Source: CAD feature listing. Evaluate the final solid. Frame: model axes, mm. A direction names the side the tool comes from. Coordinates: 2 decimals unless noted, no trailing zeros.
Item 1: Line query: probe 1 along Z at (x, y) = (60, 2); probe 2 along Z at (x, y) = (99, 2). Output: solid intervals per line, ascending.
Item 2: Pull-direction query (Z, two-part tool) for faces 3 (the cylindrical face through (78.514, 2.896, -19.391)), 4 (the flat face through (0, 3, -30)), 5 (the flat face through (141.4, 2.6, -21.4)); classes: +Z half, -Z half, draft (parallel to the pull), parting line (faces both ways), or undercut.
Item 3: Pin query (flat end, axial travel): pin 1 Ø1 at (y, z) = (2, -21.5) entering from -X; pin 2 Ø2.5 at (x, z) = (99.99, -20.02) entering from +Y (1 decimal); pin 3 Ø5.5 at (x, z) = (140, -39.99) entering from +Y. Return the tip coordinate at first contact, or that it passes through.
Item 4: Reachability of faces 1 (the cylindrical face through (141.652, 1.318, -20.411)), 2 (the cylindrical face through (122.88, 4.31, -18.5)) from +Z, -Z, +X, -X, +Y, -Y: full face, straight path, thin tool, end or side. Return the list, or none.
Item 5: Section query A-A, the plane y = 4.25. State how many separate pieces and enclosed holes the cut face has, then the cut area to 3 significant figures.
```python
from build123d import *

# Parameters (mm, degrees)
SKETCH1_W                      = 160
SKETCH1_H                      = 60
BOSS_EXTRUDE1_DEPTH            = 6
M3_CLEARANCE_HOLE1_D           = 3.4
M3_CLEARANCE_HOLE1_CSINK_D     = 3.45
M3_CLEARANCE_HOLE1_CSINK_ANGLE = 90
M3_CLEARANCE_HOLE3_D           = 3.4
M3_CLEARANCE_HOLE3_CSINK_D     = 3.45
M3_CLEARANCE_HOLE3_CSINK_ANGLE = 90
M3_CLEARANCE_HOLE4_D           = 3.2
M3_CLEARANCE_HOLE4_CSINK_D     = 3.45
M3_CLEARANCE_HOLE4_CSINK_ANGLE = 90
M3_CLEARANCE_HOLE5_D           = 3.2
M3_CLEARANCE_HOLE5_CSINK_D     = 3.45
M3_CLEARANCE_HOLE5_CSINK_ANGLE = 90
CUT_EXTRUDE3_DEPTH             = 171.985379492
CUT_EXTRUDE4_DEPTH             = 171.985379492
CUT_EXTRUDE5_DEPTH             = 171.985379492
CUT_EXTRUDE6_DEPTH             = 171.985379492
CUT_EXTRUDE7_DEPTH             = 171.985379492
CUT_EXTRUDE8_DEPTH             = 171.985379492


with BuildPart() as part:
    # Sketch1 → Boss-Extrude1 (new body)
    with BuildSketch(Plane(origin=(0, 0, 0), x_dir=(1, 0, 0), z_dir=(0, 1, 0))):
        with Locations((80, 30)):
            Rectangle(SKETCH1_W, SKETCH1_H)
    extrude(amount=BOSS_EXTRUDE1_DEPTH)

    # Sketch4 → CBORE for M3 Hex Socket Head Cap Screw1 (revolve, cut)
    with BuildSketch(Plane(origin=(139.992504276, 6, -20.042969634), x_dir=(0, 0, 1), z_dir=(1, 0, 0))):
        Polygon((0, 0), (0, 6), (1.7, 6), (1.7, 3.4), (3.25, 3.4), (3.25, 0.025), (3.275, 0), align=None)
    revolve(axis=Axis((139.992504276, 12.35, -20.042969634), (0, -1, 0)), mode=Mode.SUBTRACT)

    # Sketch7 → CBORE for M3 Hex Socket Head Cap Screw2 (revolve, cut)
    with BuildSketch(Plane(origin=(140.004074622, 6, -39.992947499), x_dir=(0, 0, 1), z_dir=(1, 0, 0))):
        Polygon((0, 0), (0, 6), (1.7, 6), (1.7, 3.4), (3.25, 3.4), (3.25, 0.025), (3.275, 0), align=None)
    revolve(axis=Axis((140.004074622, 12.35, -39.992947499), (0, -1, 0)), mode=Mode.SUBTRACT)

    # Sketch10 → CBORE for M3 Hex Socket Head Cap Screw3 (revolve, cut)
    with BuildSketch(Plane(origin=(120.000202739, 6, -39.984949452), x_dir=(0, 0, 1), z_dir=(1, 0, 0))):
        Polygon((0, 0), (0, 6), (1.6, 6), (1.6, 3.4), (3.25, 3.4), (3.25, 0.025), (3.275, 0), align=None)
    revolve(axis=Axis((120.000202739, 12.35, -39.984949452), (0, -1, 0)), mode=Mode.SUBTRACT)

    # Sketch13 → CBORE for M3 Hex Socket Head Cap Screw4 (revolve, cut)
    with BuildSketch(Plane(origin=(119.997329442, 6, -19.99932447), x_dir=(0, 0, 1), z_dir=(1, 0, 0))):
        Polygon((0, 0), (0, 6), (1.6, 6), (1.6, 3.4), (3.25, 3.4), (3.25, 0.025), (3.275, 0), align=None)
    revolve(axis=Axis((119.997329442, 12.35, -19.99932447), (0, -1, 0)), mode=Mode.SUBTRACT)

    # M3 Clearance Hole1 (through all)
    with Locations(Plane(origin=(0, 6, 0), x_dir=(1, 0, 0), z_dir=(0, 1, 0))):
        with Locations((100.019720451, 40.002637401)):
            CounterSinkHole(M3_CLEARANCE_HOLE1_D / 2, M3_CLEARANCE_HOLE1_CSINK_D / 2, counter_sink_angle=M3_CLEARANCE_HOLE1_CSINK_ANGLE)

    # M3 Clearance Hole3 (through all)
    with Locations(Plane(origin=(0, 6, 0), x_dir=(1, 0, 0), z_dir=(0, 1, 0))):
        with Locations((99.99392625, 20.015973)):
            CounterSinkHole(M3_CLEARANCE_HOLE3_D / 2, M3_CLEARANCE_HOLE3_CSINK_D / 2, counter_sink_angle=M3_CLEARANCE_HOLE3_CSINK_ANGLE)

    # M3 Clearance Hole4 (through all)
    with Locations(Plane(origin=(0, 6, 0), x_dir=(1, 0, 0), z_dir=(0, 1, 0))):
        with Locations((79.997225907, 40.005191988)):
            CounterSinkHole(M3_CLEARANCE_HOLE4_D / 2, M3_CLEARANCE_HOLE4_CSINK_D / 2, counter_sink_angle=M3_CLEARANCE_HOLE4_CSINK_ANGLE)

    # M3 Clearance Hole5 (through all)
    with Locations(Plane(origin=(0, 6, 0), x_dir=(1, 0, 0), z_dir=(0, 1, 0))):
        with Locations((79.991526723, 20.004071528)):
            CounterSinkHole(M3_CLEARANCE_HOLE5_D / 2, M3_CLEARANCE_HOLE5_CSINK_D / 2, counter_sink_angle=M3_CLEARANCE_HOLE5_CSINK_ANGLE)

    # Sketch2 → Cut-Extrude3 (cut, through all)
    with BuildSketch(Plane(origin=(0, 6, 0), x_dir=(1, 0, 0), z_dir=(0, 1, 0))):
        Polygon((61.499825244, 20.000000122), (61.29888673, 20.749912866), (60.7499125, 21.298887096), (59.999999756, 21.49982561), (59.250087012, 21.298887096), (58.701112782, 20.749912866), (58.500174268, 20.000000122), (58.701112782, 19.250087378), (59.250087012, 18.701113148), (59.999999756, 18.500174634), (60.7499125, 18.701113148), (61.29888673, 19.250087378), align=None)
    extrude(amount=-CUT_EXTRUDE3_DEPTH, mode=Mode.SUBTRACT)

    # Sketch35 → Cut-Extrude4 (cut, through all)
    with BuildSketch(Plane(origin=(0, 6, 0), x_dir=(1, 0, 0), z_dir=(0, 1, 0))):
        Polygon((58.500006975, 40), (58.700967935, 39.250003488), (59.250003488, 38.700967935), (60, 38.500006975), (60.749996512, 38.700967935), (61.299032065, 39.250003488), (61.499993025, 40), (61.299032065, 40.749996512), (60.749996512, 41.299032065), (60, 41.499993025), (59.250003488, 41.299032065), (58.700967935, 40.749996512), align=None)
    extrude(amount=-CUT_EXTRUDE4_DEPTH, mode=Mode.SUBTRACT)

    # Sketch36 → Cut-Extrude5 (cut, through all)
    with BuildSketch(Plane(origin=(0, 6, 0), x_dir=(1, 0, 0), z_dir=(0, 1, 0))):
        Polygon((41.5, 20), (41.149066665, 20.964181415), (40.260472267, 21.47721163), (39.25, 21.299038106), (38.590461069, 20.513030215), (38.590461069, 19.486969785), (39.25, 18.700961894), (40.260472267, 18.52278837), (41.149066665, 19.035818585), align=None)
    extrude(amount=-CUT_EXTRUDE5_DEPTH, mode=Mode.SUBTRACT)

    # Sketch37 → Cut-Extrude6 (cut, through all)
    with BuildSketch(Plane(origin=(0, 6, 0), x_dir=(1, 0, 0), z_dir=(0, 1, 0))):
        Polygon((41.5, 40), (41.149066665, 40.964181415), (40.260472267, 41.47721163), (39.25, 41.299038106), (38.590461069, 40.513030215), (38.590461069, 39.486969785), (39.25, 38.700961894), (40.260472267, 38.52278837), (41.149066665, 39.035818585), align=None)
    extrude(amount=-CUT_EXTRUDE6_DEPTH, mode=Mode.SUBTRACT)

    # Sketch38 → Cut-Extrude7 (cut, through all)
    with BuildSketch(Plane(origin=(0, 6, 0), x_dir=(1, 0, 0), z_dir=(0, 1, 0))):
        Polygon((21.5, 20), (20.75, 21.299038106), (19.25, 21.299038106), (18.5, 20), (19.25, 18.700961894), (20.75, 18.700961894), align=None)
    extrude(amount=-CUT_EXTRUDE7_DEPTH, mode=Mode.SUBTRACT)

    # Sketch39 → Cut-Extrude8 (cut, through all)
    with BuildSketch(Plane(origin=(0, 6, 0), x_dir=(1, 0, 0), z_dir=(0, 1, 0))):
        Polygon((21.5, 40), (20.75, 41.299038106), (19.25, 41.299038106), (18.5, 40), (19.25, 38.700961894), (20.75, 38.700961894), align=None)
    extrude(amount=-CUT_EXTRUDE8_DEPTH, mode=Mode.SUBTRACT)


solid = part.part
```
Verdict:
1. probe 1: z = -60 to -41.5, -38.5 to -21.5, -18.5 to 0
1. probe 2: z = -60 to -41.36, -38.64 to -21.4, -18.64 to 0
2. face 3: undercut
2. face 4: draft
2. face 5: undercut
3. pin 1: stops at x = 0
3. pin 2: passes through
3. pin 3: stops at y = 2.6
4. face 1: +Y, -Y
4. face 2: +Y
5. separate pieces: 1
5. enclosed holes: 14
5. area: 9,390 mm2
